The listing builds one solid part. Answer for the finished solid, in the listing's coordinates (mm). A direction names the side the tool comes from. Give positions to 0.01 mm unless a question says otherwise; leave off trailing zeros. Order: outer loops, then holes, each group sorted by start corner. A loop starts at its lowest first (then second) coordinate and runs counter-clockwise, first axis right, second up. Notation, with made-up numbers: (14, -39) - (42, -39) arc R16 cw to (42, -28) - close; hole circle Ø6 at (-27, 3). An arc over 180 degrees is marked (long way). Write each question's results on one line, items separated by ' | '. Start each with the question number.
1. Flat-ended cylindrical pins translate along their axes: pin 1 (6 mm diameter, centred on y = -3.5, z = -27, fed in from +X); pin 2 (2 mm diameter, centred on x = 60, y = 20.5, fed in from +Z); pin 3 (6 mm diameter, centred on y = -7.5, z = -26.5, fed in from +X). Find the tip coordinate at first contact, or state that the pin passes through.
2. Section D-D (y = 28.5) is taken. Give the vertices of the cut face in (x, z).
3. Section A-A (y = 0) is taken. Give the vertices of the cut face in (x, z).
4. Which of the six approach directions +Z, -Z, +X, -X, +Y, -Y give full straight-line access (tool end or side, diameter ignored) to faces 1 (the face through (59.3, 20.66, -13.17)), 2 (the face through (113.521, 7.509, -23.846)), 3 (the face through (0, 1, 1))?
5. Section C-C (x = 60) is taken. Give the vertices of the cut face in (y, z), and give its area (3 significant figures).
6. Find the intervals of material crossed by L1, parallel to X at y = 32.5, z = -6; L2, parallel to X at y = -11, z = -20; L3, parallel to X at y = 10.5, z = -20, in increasing order.
7. Determine the mould class of faces 4 (the face through (112, 3.82, 22.34)), 5 (the face through (110, -20, -11)), 6 (the face through (4.93, 37.18, 4.88)), 7 (the face through (120, 0, 0)) for opening direction X: released by +X, released by -X, zero draft, split by the parting line, or undercut.
from build123d import *

# Parameters (mm, degrees)
SKETCH1_R          = 37.5
EXTRUDE1_DEPTH     = 10
SKETCH2_R          = 24.5
EXTRUDE2_DEPTH     = 110
SKETCH3_OUTSIDE_W  = 109.032
SKETCH3_OUTSIDE_H  = 109.032
SKETCH3_OUTSIDE_R  = 22.5
CUT_EXTRUDE1_DEPTH = 10
SKETCH4_R          = 25
EXTRUDE3_DEPTH     = 8
CHAMFER1_SIZE      = 5


with BuildPart() as part:
    # Sketch1 → Extrude1 (new body)
    with BuildSketch(Plane(origin=(0, 0, 0), x_dir=(0, 0, -1), z_dir=(1, 0, 0))):
        Circle(SKETCH1_R)
    extrude(amount=EXTRUDE1_DEPTH)

    # Sketch2 → Extrude2 (add)
    with BuildSketch(Plane(origin=(10, 0, 0), x_dir=(0, 0, -1), z_dir=(1, 0, 0))):
        Circle(SKETCH2_R)
    extrude(amount=EXTRUDE2_DEPTH)

    # Sketch3 outside → Cut-Extrude1 (cut)
    with BuildSketch(Plane(origin=(120, 0, 0), x_dir=(0, 0, -1), z_dir=(1, 0, 0))):
        Rectangle(SKETCH3_OUTSIDE_W, SKETCH3_OUTSIDE_H)
        Circle(SKETCH3_OUTSIDE_R, mode=Mode.SUBTRACT)
    extrude(amount=-CUT_EXTRUDE1_DEPTH, mode=Mode.SUBTRACT)

    # Sketch4 → Extrude3 (add)
    with BuildSketch(Plane(origin=(120, 0, 0), x_dir=(0, 0, -1), z_dir=(1, 0, 0))):
        Circle(SKETCH4_R)
    extrude(amount=-EXTRUDE3_DEPTH)

    # Chamfer1
    chamfer1_edges = [part.edges().sort_by_distance(p)[0] for p in [
        (120, 0, 25),
    ]]
    chamfer(chamfer1_edges, length=CHAMFER1_SIZE)


solid = part.part
Reported:
1) pin 1: x = 115.77 | pin 2: z = 14.83 | pin 3: x = 115.46
2) outline: (0, -24.37) - (10, -24.37) - (10, 24.37) - (0, 24.37) - close
3) outline: (0, -37.5) - (10, -37.5) - (10, -24.5) - (110, -24.5) - (110, -22.5) - (112, -22.5) - (112, -25) - (115, -25) - (120, -20) - (120, 20) - (115, 25) - (112, 25) - (112, 22.5) - (110, 22.5) - (110, 24.5) - (10, 24.5) - (10, 37.5) - (0, 37.5) - close
4) face 1: none | face 2: +X | face 3: +Z, -Z, -X, +Y, -Y
5) outline: circle Ø49 at (0, 0) | area: 1,890 mm²
6) L1: 0 to 10 | L2: 0 to 110, 112 to 117.17 | L3: 0 to 110, 112 to 117.41
7) face 4: undercut | face 5: undercut | face 6: zero draft | face 7: released by +X
